from build123d import *

# Parameters (mm, degrees)
SKETCH1_W           = 15
SKETCH1_H           = 15
SKETCH1_W_2         = 11
SKETCH1_H_2         = 11
BOSS_EXTRUDE1_DEPTH = 245
SKETCH2_R           = 1.6
CUT_EXTRUDE1_DEPTH  = 246.916652547
SKETCH4_R           = 2.6
CUT_EXTRUDE2_DEPTH  = 246.916652547
SKETCH5_R           = 1.6
CUT_EXTRUDE3_DEPTH  = 246.916652547


with BuildPart() as part:
    # Sketch1 → Boss-Extrude1 (new body)
    with BuildSketch(Plane(origin=(0, 0, 0), x_dir=(1, 0, 0), z_dir=(0, 1, 0))):
        with Locations((7.5, 7.5)):
            Rectangle(SKETCH1_W, SKETCH1_H)
        with Locations((7.5, 7.5)):
            Rectangle(SKETCH1_W_2, SKETCH1_H_2, mode=Mode.SUBTRACT)
    extrude(amount=BOSS_EXTRUDE1_DEPTH)

    # Sketch2 → Cut-Extrude1 (cut, through all)
    with BuildSketch(Plane(origin=(15, 0, 0), x_dir=(0, 0, -1), z_dir=(1, 0, 0))):
        with Locations((7.5, 215)):
            Circle(SKETCH2_R)
        with Locations((7.5, 205)):
            Circle(SKETCH2_R)
        with Locations((7.5, 30)):
            Circle(SKETCH2_R)
        with Locations((7.5, 40)):
            Circle(SKETCH2_R)
    extrude(amount=-CUT_EXTRUDE1_DEPTH, mode=Mode.SUBTRACT)

    # Sketch4 → Cut-Extrude2 (cut, through all)
    with BuildSketch(Plane(origin=(0, 0, -15), x_dir=(-1, 0, 0), z_dir=(0, 0, -1))):
        with Locations((-7.5, 235)):
            Circle(SKETCH4_R)
        with Locations((-7.5, 225)):
            Circle(SKETCH4_R)
        with Locations((-7.5, 10)):
            Circle(SKETCH4_R)
        with Locations((-7.5, 20)):
            Circle(SKETCH4_R)
    extrude(amount=-CUT_EXTRUDE2_DEPTH, mode=Mode.SUBTRACT)

    # Sketch5 → Cut-Extrude3 (cut, through all)
    with BuildSketch(Plane(origin=(0, 0, -15), x_dir=(-1, 0, 0), z_dir=(0, 0, -1))):
        with Locations((-7.5, 45)):
            Circle(SKETCH5_R)
        with Locations((-7.5, 75)):
            Circle(SKETCH5_R)
        with Locations((-7.5, 200)):
            Circle(SKETCH5_R)
        with Locations((-7.5, 170)):
            Circle(SKETCH5_R)
        with Locations((-7.5, 140)):
            Circle(SKETCH5_R)
        with Locations((-7.5, 105)):
            Circle(SKETCH5_R)
    extrude(amount=-CUT_EXTRUDE3_DEPTH, mode=Mode.SUBTRACT)


solid = part.part
Can you work these out from the model? Positions are in its coordinate system, mm. A direction names the side the tool comes from. Coordinates: 2 decimals unless noted, no trailing zeros. Write each loop counter-clockwise with the first axis right and the second up, starting at its lowest first coordinate (ties: lowest second). Pieces come first, ordered by that corner, then holes.
Q1. If we mould it in two halves opening along Z, with no side actions, what happens to faces 3 (the face through (7, 121, -2)), 4 (the face through (7, 121, -15)), 5 (the face through (6.3, 7.693, -1.014)), 6 (the face through (7, 121, 0))? For each: +Z half, -Z half, draft (parallel to the pull), parting line (faces both ways), or undercut.
Results found:
face 3: undercut
face 4: -Z half
face 5: draft
face 6: +Z half
Q2. Please list where these lines run through material, in increasing order: L1, parallel to Y at x = 0.4, z = -7.5; L2, parallel to Z at x = 9.5, y = 74.5; L3, parallel to X at y = 200, z = -1.3.
Results found:
L1: y = 0 to 28.4, 31.6 to 38.4, 41.6 to 203.4, 206.6 to 213.4, 216.6 to 245
L2: z = -15 to -13, -2 to 0
L3: x = 0 to 5.9, 9.1 to 15
Q3. Imagine slicing it at B-B, the plane y = 20. List the corners of the cut face in (x, z) for me, plus the area to 3 significant figures.
Results found:
outline: (0, -15) - (4.9, -15) - (4.9, -13) - (2, -13) - (2, -2) - (4.9, -2) - (4.9, 0) - (0, 0) - close; (10.1, -15) - (15, -15) - (15, 0) - (10.1, 0) - (10.1, -2) - (13, -2) - (13, -13) - (10.1, -13) - close
area: 83.2 mm2
Q4. For P1, Ø3, axis at y = 30, z = -7.5, coming from the -X side, with a flat end and sliding along its axis, tell me the tip position at first contact or that it passes through.
Results found:
P1: passes through
Q5. Imagine slicing it at A-A, the plane y = 146. List the corners of the cut face in (x, z) for me.
Results found:
outline: (0, -15) - (15, -15) - (15, 0) - (0, 0) - close; hole (2, -13) - (13, -13) - (13, -2) - (2, -2) - close
Q6. Which directions (+Z, -Z, +X, -X, +Y, -Y) give clear straight access to the entire face, cutting with the end or side of a thin tool? Please do faces 1 (the face through (7.838, 237.578, -14.014)), 2 (the face through (2, 121, -7)).
Results found:
face 1: +Z, -Z
face 2: +Y, -Y
